The listing builds one solid part. Answer for the finished solid, in the listing's coordinates (mm). Coordinates: 2 decimals unless noted, no trailing zeros. Order: outer loops, then holes, each group sorted by start corner. A loop starts at its lowest first (then second) coordinate and runs counter-clockwise, first axis right, second up. Notation, with made-up numbers: (0, 30) -> (39, 30) arc R30 cw to (39, 55) -> close; hole circle Ø5 at (20, -25.5). An arc over 180 degrees is marked (long way). Write item = value, one per line.
from build123d import *

# Parameters (mm, degrees)
BOSS_EXTRUDE2_DEPTH = 3.175
BOSS_EXTRUDE3_DEPTH = 3.175
BOSS_EXTRUDE8_DEPTH = 3.175
SKETCH12_W          = 70.49262
SKETCH12_H          = 3.175
BOSS_EXTRUDE9_DEPTH = 3.175
SKETCH15_R          = 2.25
CUT_EXTRUDE1_DEPTH  = 371.49176257
SKETCH16_R          = 2.250000072
SKETCH16_R_2        = 2.25
CUT_EXTRUDE2_DEPTH  = 371.49176257


with BuildPart() as part:
    # Sketch1 → Boss-Extrude2 (new body)
    with BuildSketch(Plane.XY):
        Polygon((129.013076168, 254.245404572), (-18.685383832, 254.245404572), (-18.685383832, 157.666984572), (92.088461168, 157.666984572), (92.088461168, 154.491984572), (-18.685383832, 154.491984572), (-18.685383832, 57.913564572), (92.088461168, 57.913564572), (92.088461168, 54.738564572), (-18.685383832, 54.738564572), (-18.685383832, -41.839855428), (92.088461168, -41.839855428), (92.088461168, -45.014855428), (-18.685383832, -45.014855428), (-18.685383832, -141.593275428), (92.088461168, -141.593275428), (92.088461168, -144.768275428), (-18.685383832, -144.768275428), (-18.685383832, -241.346695428), (129.013076168, -241.346695428), align=None)
    extrude(amount=BOSS_EXTRUDE2_DEPTH)

    # Sketch4 → Boss-Extrude3 (add, through all)
    with BuildSketch(Plane.XY.offset(3.175)):
        Polygon((129.013076168, 254.245404572), (129.013076168, -241.346695428), (153.407236168, -241.346695428), (153.407236168, -227.262720585), (153.407236168, 240.16142973), (153.407236168, 254.245404572), align=None)
    extrude(amount=-BOSS_EXTRUDE3_DEPTH)

    # Sketch11 → Boss-Extrude8 (add, through all)
    with BuildSketch(Plane.XY.offset(3.175)):
        Polygon((266.437236168, 134.679984572), (266.437236168, 54.738564572), (153.407236168, 54.738564572), (153.407236168, 134.679984572), (153.407236168, 254.245404572), align=None)
    extrude(amount=-BOSS_EXTRUDE8_DEPTH)

    # Sketch12 → Boss-Extrude9 (add, through all)
    with BuildSketch(Plane(origin=(0, 0, 0), x_dir=(-1, 0, 0), z_dir=(0, 0, -1))):
        with Locations((-16.560926168, 255.832904572)):
            Rectangle(SKETCH12_W, SKETCH12_H)
        with Locations((-16.560926168, -242.934195428)):
            Rectangle(SKETCH12_W, SKETCH12_H)
    extrude(amount=-BOSS_EXTRUDE9_DEPTH)

    # Sketch15 → Cut-Extrude1 (cut, through all)
    with BuildSketch(Plane.XY.offset(3.175)):
        with Locations((143.247236168, 231.313297791)):
            Circle(SKETCH15_R)
        with Locations((143.247236168, 164.651984572)):
            Circle(SKETCH15_R)
        with Locations((255.799716168, 113.343984572)):
            Circle(SKETCH15_R)
        with Locations((255.799716168, 74.495671354)):
            Circle(SKETCH15_R)
        with Locations((143.247236168, 29.338564572)):
            Circle(SKETCH15_R)
        with Locations((143.247236168, -32.334232694)):
            Circle(SKETCH15_R)
        with Locations((143.247236168, -94.538012037)):
            Circle(SKETCH15_R)
        with Locations((143.247236168, -156.74179138)):
            Circle(SKETCH15_R)
        with Locations((143.247236168, -218.414588646)):
            Circle(SKETCH15_R)
    extrude(amount=-CUT_EXTRUDE1_DEPTH, mode=Mode.SUBTRACT)

    # Sketch16 → Cut-Extrude2 (cut, through all)
    with BuildSketch(Plane.XY.offset(3.175)):
        with Locations((138.792076168, 121.451235566)):
            Circle(SKETCH16_R)
        with Locations((138.792076168, 82.140925566)):
            Circle(SKETCH16_R_2)
    extrude(amount=-CUT_EXTRUDE2_DEPTH, mode=Mode.SUBTRACT)


solid = part.part
Q1. Each of these flat-tipped pins is pushed along its axis until it touches: pin 1 Ø2.5 at (x, y) = (143.25, 231.31) entering from -Z; pin 2 Ø1 at (y, z) = (-42.5, 2) entering from -X; pin 3 Ø1.5 at (y, z) = (22.5, 2.5) entering from +X. Where does it stop, or does it pass through?
The answers:
pin_1 = through
pin_2 = 92.09
pin_3 = 153.41
Q2. Section C-C, the plane y = -15.5 is taken. Give the vertices of the cut face in (x, z) (3 decimals).
The answers:
outline = (-18.685, 0) -> (153.407, 0) -> (153.407, 3.175) -> (-18.685, 3.175) -> close
Q3. Section A-A, the plane x = 59.5 is taken. Give the vertices of the cut face in (y, z) (3 decimals).
The answers:
outline = (-241.347, 0) -> (-144.768, 0) -> (-144.768, 3.175) -> (-241.347, 3.175) -> close; (-141.593, 0) -> (-45.015, 0) -> (-45.015, 3.175) -> (-141.593, 3.175) -> close; (-41.84, 0) -> (54.739, 0) -> (54.739, 3.175) -> (-41.84, 3.175) -> close; (57.914, 0) -> (154.492, 0) -> (154.492, 3.175) -> (57.914, 3.175) -> close; (157.667, 0) -> (254.245, 0) -> (254.245, 3.175) -> (157.667, 3.175) -> close
Q4. Section B-B, the plane x = 19.5 is taken. Give the vertices of the cut face in (y, z) (3 decimals), plus the area to 3 significant figures.
The answers:
outline = (-244.522, 0) -> (-144.768, 0) -> (-144.768, 3.175) -> (-244.522, 3.175) -> close; (-141.593, 0) -> (-45.015, 0) -> (-45.015, 3.175) -> (-141.593, 3.175) -> close; (-41.84, 0) -> (54.739, 0) -> (54.739, 3.175) -> (-41.84, 3.175) -> close; (57.914, 0) -> (154.492, 0) -> (154.492, 3.175) -> (57.914, 3.175) -> close; (157.667, 0) -> (257.42, 0) -> (257.42, 3.175) -> (157.667, 3.175) -> close
area = 1,550 mm2
Q5. Find the intervals of material crossed by line 1 along Y through (x, z) = (82.5, 1); line 2 along Y through (x, z) = (25.5, 1.35); line 3 along X through (y, z) = (82.5, 1.6), in increasing order.
The answers:
line_1 = -241.35 to -144.77, -141.59 to -45.01, -41.84 to 54.74, 57.91 to 154.49, 157.67 to 254.25
line_2 = -244.52 to -144.77, -141.59 to -45.01, -41.84 to 54.74, 57.91 to 154.49, 157.67 to 257.42
line_3 = -18.69 to 136.57, 141.01 to 266.44
Q6. Section D-D, the plane z = 2.35 is taken. Give the number of separate pieces and of enclosed holes in the cut face, plus the area to 3 significant figures.
The answers:
separate_pieces = 1
enclosed_holes = 11
area = 99,900 mm2
